Build history of the part. All positions in model axes, mm. Face numbers are marked on the shaded views. A direction names the side the tool comes from. Give positions to 0.01 mm unless a question says otherwise; leave off trailing zeros. Loops run counter-clockwise (first coordinate to the right, second up) from the corner with the lowest first, then second, coordinate; pieces in that order, holes last. Notation, with made-up numbers: M 63.25,42 L 120.25,42 A23 cw 120.25,66 Z; hole C 85.25,-32 d2. An arc over 180 degrees is marked long. Put each result on its own line as item: value.
```python
from build123d import *

# Parameters (mm, degrees)
SKETCH1_R            = 2.25
BOSS_EXTRUDE1_DEPTH  = 20
SKETCH2_R            = 2.25
BOSS_EXTRUDE2_DEPTH  = 10
SKETCH4_W            = 26.5
SKETCH4_H            = 2.5
CUT_EXTRUDE1_DEPTH   = 39.17921555
CHAMFER2_SIZE        = 4
CHAMFER3_SIZE        = 4
FILLET4_R            = 2
SKETCH7_W            = 10
SKETCH7_H            = 10
BOSS_EXTRUDE5_DEPTH  = 20
FILLET6_R            = 2
SKETCH8_W            = 63
SKETCH8_H            = 30
BOSS_EXTRUDE6_DEPTH  = 4
CHAMFER4_SIZE        = 2
FILLET7_R            = 2
SKETCH13_R           = 2.25
BOSS_EXTRUDE8_DEPTH  = 20
CUT_EXTRUDE2_DEPTH   = 54.816005983
BOSS_EXTRUDE9_START  = -10
SKETCH14_R           = 2.25
BOSS_EXTRUDE9_DEPTH  = 10
SKETCH15_R           = 2.25
BOSS_EXTRUDE10_DEPTH = 0.4


with BuildPart() as part:
    # Sketch1 → Boss-Extrude1 (new body)
    with BuildSketch(Plane(origin=(0, 0, 0), x_dir=(0, 0, -1), z_dir=(1, 0, 0))):
        Polygon((10.25, -20.3), (13.25, -20.3), (13.25, 29.7), (-13.25, 29.7), (-13.25, -20.3), (-10.25, -20.3), (-10.25, 20.3), (10.25, 20.3), align=None)
        with Locations((5, 24)):
            Circle(SKETCH1_R, mode=Mode.SUBTRACT)
        with Locations((-5, 24)):
            Circle(SKETCH1_R, mode=Mode.SUBTRACT)
    extrude(amount=BOSS_EXTRUDE1_DEPTH)

    # Sketch2 → Boss-Extrude2 (add)
    with BuildSketch(Plane.ZY):
        with Locations((-5, 24)):
            Circle(SKETCH2_R)
        with Locations((5, 24)):
            Circle(SKETCH2_R)
    extrude(amount=-BOSS_EXTRUDE2_DEPTH)

    # Sketch4 → Cut-Extrude1 (cut, through all)
    with BuildSketch(Plane(origin=(20, 0, 0), x_dir=(0, 0, -1), z_dir=(1, 0, 0))):
        with Locations((0, 28.45)):
            Rectangle(SKETCH4_W, SKETCH4_H)
    extrude(amount=-CUT_EXTRUDE1_DEPTH, mode=Mode.SUBTRACT)

    # Chamfer2
    chamfer2_edges = [part.edges().sort_by_distance(p)[0] for p in [
        (10, 27.2, -13.25),
    ]]
    chamfer(chamfer2_edges, length=CHAMFER2_SIZE)

    # Chamfer3
    chamfer3_edges = [part.edges().sort_by_distance(p)[0] for p in [
        (10, 27.2, 13.25),
    ]]
    chamfer(chamfer3_edges, length=CHAMFER3_SIZE)

    # Fillet4
    fillet4_edges = [part.edges().sort_by_distance(p)[0] for p in [
        (10, 27.2, -9.25),
        (10, 27.2, 9.25),
    ]]
    fillet(fillet4_edges, radius=FILLET4_R)

    # Sketch7 → Boss-Extrude5 (add)
    with BuildSketch(Plane(origin=(20, 0, 0), x_dir=(0, 0, -1), z_dir=(1, 0, 0))):
        with Locations((18.25, -0.3)):
            Rectangle(SKETCH7_W, SKETCH7_H)
    extrude(amount=-BOSS_EXTRUDE5_DEPTH)

    # Fillet6
    fillet6_edges = [part.edges().sort_by_distance(p)[0] for p in [
        (10, -5.3, -13.25),
        (10, 4.7, -13.25),
    ]]
    fillet(fillet6_edges, radius=FILLET6_R)

    # Sketch8 → Boss-Extrude6 (add)
    with BuildSketch(Plane(origin=(0, 0, -23.25), x_dir=(-1, 0, 0), z_dir=(0, 0, -1))):
        with Locations((-13.9, -0.3)):
            Rectangle(SKETCH8_W, SKETCH8_H)
    extrude(amount=BOSS_EXTRUDE6_DEPTH)

    # Chamfer4
    chamfer4_edges = [part.edges().sort_by_distance(p)[0] for p in [
        (45.4, -0.3, -23.25),
        (13.9, -15.3, -23.25),
        (-17.6, -0.3, -23.25),
        (13.9, 14.7, -23.25),
    ]]
    chamfer(chamfer4_edges, length=CHAMFER4_SIZE)

    # Fillet7
    fillet7_edges = [part.edges().sort_by_distance(p)[0] for p in [
        (10, 4.7, -23.25),
        (10, -5.3, -23.25),
    ]]
    fillet(fillet7_edges, radius=FILLET7_R)

    # Sketch13 → Boss-Extrude8 (add)
    with BuildSketch(Plane(origin=(20, 0, 0), x_dir=(0, 0, -1), z_dir=(1, 0, 0))):
        with BuildLine():
            Line((-13.25, -23.2), (-9.835786438, -26.614213562))
            ThreePointArc((-9.835786438, -26.614213562), (-9.18693974, -27.047759065), (-8.421572875, -27.2))
            Line((-8.421572875, -27.2), (8.421572875, -27.2))
            ThreePointArc((8.421572875, -27.2), (9.18693974, -27.047759065), (9.835786438, -26.614213562))
            Line((9.835786438, -26.614213562), (13.25, -23.2))
            Line((13.25, -23.2), (13.25, -20.3))
            Line((13.25, -20.3), (-13.25, -20.3))
            Line((-13.25, -20.3), (-13.25, -23.2))
        make_face()
        with Locations((5, -24)):
            Circle(SKETCH13_R, mode=Mode.SUBTRACT)
        with Locations((-5, -24)):
            Circle(SKETCH13_R, mode=Mode.SUBTRACT)
    extrude(amount=-BOSS_EXTRUDE8_DEPTH)

    # Sketch12 → Cut-Extrude2 (cut, through all)
    with BuildSketch(Plane(origin=(20, 0, 0), x_dir=(0, 0, -1), z_dir=(1, 0, 0))):
        with BuildLine():
            Line((13.25, 23.2), (9.835786438, 26.614213562))
            ThreePointArc((9.835786438, 26.614213562), (9.18693974, 27.047759065), (8.421572875, 27.2))
            Line((8.421572875, 27.2), (-8.421572875, 27.2))
            ThreePointArc((-8.421572875, 27.2), (-9.18693974, 27.047759065), (-9.835786438, 26.614213562))
            Line((-9.835786438, 26.614213562), (-13.25, 23.2))
            Line((-13.25, 23.2), (-13.25, 20.3))
            Line((-13.25, 20.3), (13.25, 20.3))
            Line((13.25, 20.3), (13.25, 23.2))
        make_face()
    extrude(amount=-CUT_EXTRUDE2_DEPTH, mode=Mode.SUBTRACT)

    # Sketch14 → Boss-Extrude9 (add)
    with BuildSketch(Plane.ZY.offset(BOSS_EXTRUDE9_START)):
        with Locations(Location((-5, -24, 0), (0, 0, 180))):
            Circle(SKETCH14_R)
        with Locations(Location((5, -24, 0), (0, 0, 180))):
            Circle(SKETCH14_R)
    extrude(amount=BOSS_EXTRUDE9_DEPTH)

    # Sketch15 → Boss-Extrude10 (add)
    with BuildSketch(Plane(origin=(20, 0, 0), x_dir=(0, 0, -1), z_dir=(1, 0, 0))):
        with BuildLine():
            Line((-10.25, 20.3), (-13.25, 20.3))
            Line((-13.25, 20.3), (-13.25, -23.2))
            Line((-13.25, -23.2), (-9.835786438, -26.614213562))
            ThreePointArc((-9.835786438, -26.614213562), (-9.18693974, -27.047759065), (-8.421572875, -27.2))
            Line((-8.421572875, -27.2), (8.421572875, -27.2))
            ThreePointArc((8.421572875, -27.2), (9.18693974, -27.047759065), (9.835786438, -26.614213562))
            Line((9.835786438, -26.614213562), (13.25, -23.2))
            Line((13.25, -23.2), (13.25, -7.3))
            ThreePointArc((13.25, -7.3), (13.835786438, -5.885786438), (15.25, -5.3))
            Line((15.25, -5.3), (21.25, -5.3))
            ThreePointArc((21.25, -5.3), (22.664213562, -5.885786438), (23.25, -7.3))
            Line((23.25, -7.3), (23.25, 6.7))
            ThreePointArc((23.25, 6.7), (22.664213562, 5.285786438), (21.25, 4.7))
            Line((21.25, 4.7), (15.25, 4.7))
            ThreePointArc((15.25, 4.7), (13.835786438, 5.285786438), (13.25, 6.7))
            Line((13.25, 6.7), (13.25, 20.3))
            Line((13.25, 20.3), (10.25, 20.3))
            Line((10.25, 20.3), (10.25, -20.3))
            Line((10.25, -20.3), (-10.25, -20.3))
            Line((-10.25, -20.3), (-10.25, 20.3))
        make_face()
        with Locations((5, -24)):
            Circle(SKETCH15_R, mode=Mode.SUBTRACT)
        with Locations((-5, -24)):
            Circle(SKETCH15_R, mode=Mode.SUBTRACT)
    extrude(amount=BOSS_EXTRUDE10_DEPTH)


solid = part.part
```
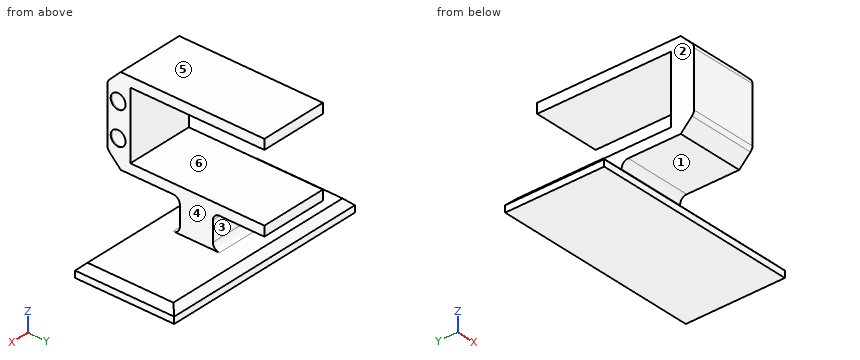
Q1. Mould opens along Z. For the marked faces 4, 5 and 6 say: pulls with the +Z half, pulls with the -Z half, needs draft (parallel to the pull), parting line crosses it, or undercut.
Here are the results:
face 4: needs draft
face 5: pulls with the +Z half
face 6: undercut
Q2. Drop flat-ended pins along their axis: pin 1 Ø6.5 at (x, z) = (9, -18) entering from -Y; pin 2 Ø5 at (y, z) = (-25, -4) entering from +X; pin 3 Ø6 at (y, z) = (-24, -5) entering from -X; pin 4 Ø10 at (x, z) = (31.5, -17) entering from +Y. Give the stop position or say it passes through.
Here are the results:
pin 1: y = -5.36
pin 2: x = 20.4
pin 3: x = 0
pin 4: through
Q3. Slice it at A-A (y = 7.5). List the corners of the cut face in (x, z).
Here are the results:
outline: M -17.6,-27.25 L 45.4,-27.25 L 45.4,-25.25 L 43.4,-23.25 L -15.6,-23.25 L -17.6,-25.25 Z; M 0,-13.25 L 20.4,-13.25 L 20.4,-10.25 L 0,-10.25 Z; M 0,10.25 L 20.4,10.25 L 20.4,13.25 L 0,13.25 Z
Q4. Slice it at B-B (z = 5). List the corners of the cut face in (x, y).
Here are the results:
outline: M 0,-27.2 L 20.4,-27.2 L 20.4,-26.25 L 10,-26.25 L 10,-21.75 L 20.4,-21.75 L 20.4,-20.3 L 0,-20.3 Z
Q5. Slice it at D-D (x = 7.5). List the corners of the cut face in (y, z).
Here are the results:
outline: M -27.2,-8.42 A2 ccw -26.61,-9.84 L -23.2,-13.25 L -7.3,-13.25 A2 cw -5.3,-15.25 L -5.3,-21.25 A2 cw -7.3,-23.25 L -13.3,-23.25 L -15.3,-25.25 L -15.3,-27.25 L 14.7,-27.25 L 14.7,-25.25 L 12.7,-23.25 L 6.7,-23.25 A2 cw 4.7,-21.25 L 4.7,-15.25 A2 cw 6.7,-13.25 L 20.3,-13.25 L 20.3,-10.25 L -20.3,-10.25 L -20.3,10.25 L 20.3,10.25 L 20.3,13.25 L -23.2,13.25 L -26.61,9.84 A2 ccw -27.2,8.42 Z
Q6. Slice it at C-C (y = -24). List the corners of the cut face in (x, z), and give its area (3 significant figures).
Here are the results:
outline: M 0,-12.45 L 20.4,-12.45 L 20.4,-7.25 L 10,-7.25 L 10,-2.75 L 20.4,-2.75 L 20.4,2.75 L 10,2.75 L 10,7.25 L 20.4,7.25 L 20.4,12.45 L 0,12.45 Z
area: 414 mm²
Q7. Probe line 1 (Z direction, x = 11.5, y = 11); line 2 (Y direction, x = 12.5, z = -5); line 3 (Z direction, x = 15.5, y = -5). List the from-to ranges inside material, lowest first. Write a range as from..to.
Here are the results:
line 1: -27.25..-23.25, -13.25..-10.25, 10.25..13.25
line 2: -27.2..-26.25, -21.75..-20.3
line 3: -27.25..-10.25, 10.25..13.25
Q8. Tool access for the marked faces 1, 2 and 3: list every direction of +Z, -Z, +X, -X, +Y, -Y with a clear straight run to the whole face (end or side of a thin tool).
Here are the results:
face 1: +X, -X, -Y
face 2: +Z, -X, +Y, -Y
face 3: +X, -X, +Y
